Print and shaded views of the part. All mm, measured from the part's lowest x, y and z. A direction names the side the tool comes from. Coordinates: 2 decimals unless noted, no trailing zeros. Write each loop counter-clockwise with the first axis right and the second up, starting at its lowest first coordinate (ties: lowest second). Pieces come first, ordered by that corner, then holes. Notation, with made-up numbers: (-4.5, 84) -> (12.5, 84) arc R13 cw to (12.5, 108) -> close; hole circle Ø3 at (-0.5, 58). An arc over 180 degrees is marked (long way). Write item = value, one per line.
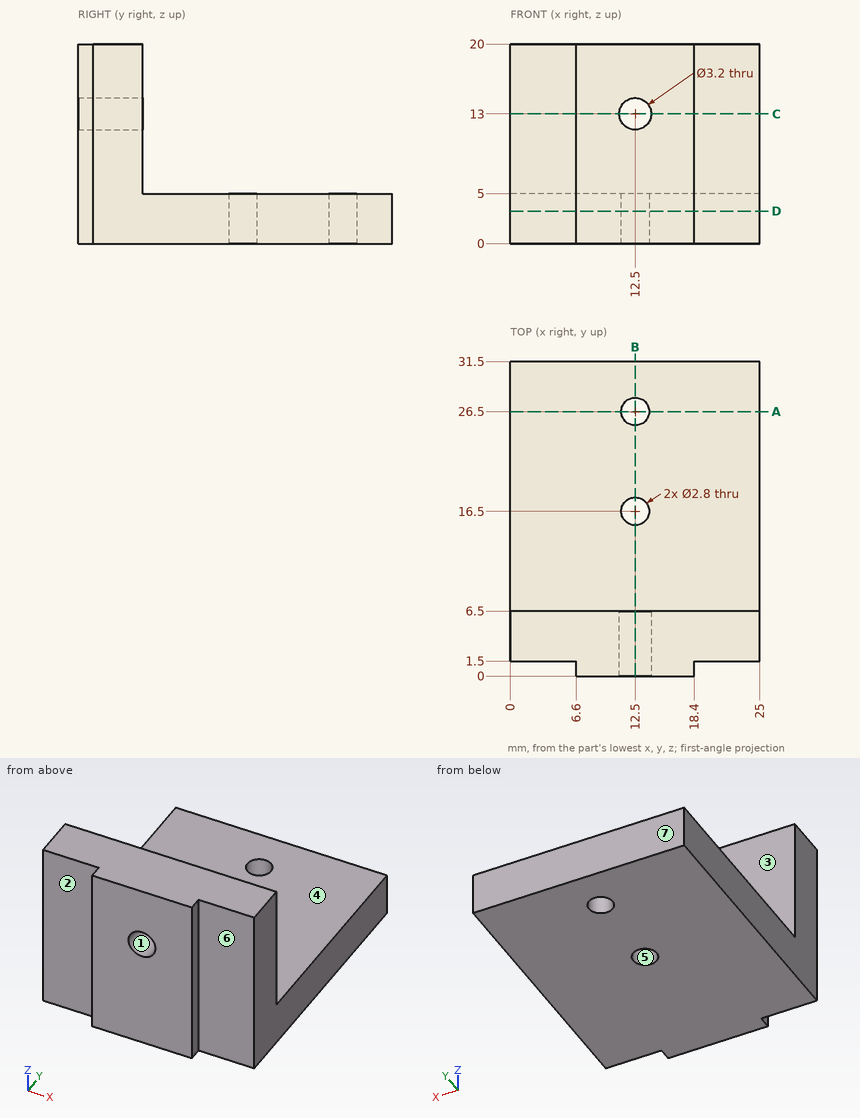
Q1. Saw through at A-A on y = 26.5. Give the cut face in (x, z), and give its area (3 significant figures).
Model answer:
outline = (0, 0) -> (11.1, 0) -> (11.1, 5) -> (0, 5) -> close; (13.9, 0) -> (25, 0) -> (25, 5) -> (13.9, 5) -> close
area = 111 mm²
Q2. Saw through at B-B on x = 12.5. Give the cut face in (y, z).
Model answer:
outline = (0, 0) -> (15.1, 0) -> (15.1, 5) -> (6.5, 5) -> (6.5, 11.4) -> (0, 11.4) -> close; (0, 14.6) -> (6.5, 14.6) -> (6.5, 20) -> (0, 20) -> close; (17.9, 0) -> (25.1, 0) -> (25.1, 5) -> (17.9, 5) -> close; (27.9, 0) -> (31.5, 0) -> (31.5, 5) -> (27.9, 5) -> close
Q3. Saw through at C-C on z = 13. Give the cut face in (x, y), and give its area (3 significant figures).
Model answer:
outline = (0, 1.5) -> (6.6, 1.5) -> (6.6, 0) -> (10.9, 0) -> (10.9, 6.5) -> (0, 6.5) -> close; (14.1, 0) -> (18.4, 0) -> (18.4, 1.5) -> (25, 1.5) -> (25, 6.5) -> (14.1, 6.5) -> close
area = 122 mm²
Q4. Mould opens along Y. For the marked faces 4, 5, 6 and 7 say: released by +Y, released by -Y, zero draft, split by the parting line, or undercut.
Model answer:
face_4 = zero draft
face_5 = undercut
face_6 = released by -Y
face_7 = released by +Y
Q5. Which spindle directions (+Z, -Z, +X, -X, +Y, -Y) get a long thin tool onto all of the face, cutting with end or side? Do the marked faces 1, 2 and 3. Say none if no direction does.
Model answer:
face_1 = +Y, -Y
face_2 = +Z, -Z, -X, -Y
face_3 = +Z, +X, -X, +Y
Q6. Pin check, flat tips, straight feed: pin 1 (4.5 mm diameter, centred on x = 12.5, y = 16.5, fed in from +Z); pin 2 (7.5 mm diameter, centred on x = 10, z = 14.5, fed in from +Y); pin 3 (5.5 mm diameter, centred on x = 22, z = 8, fed in from -Y). Stop position of each tip, or through.
Model answer:
pin_1 = 5
pin_2 = 6.5
pin_3 = 1.5
Q7. Saw through at D-D on z = 3.25. Give the cut face in (x, y).
Model answer:
outline = (0, 1.5) -> (6.6, 1.5) -> (6.6, 0) -> (18.4, 0) -> (18.4, 1.5) -> (25, 1.5) -> (25, 31.5) -> (0, 31.5) -> close; hole circle Ø2.8 at (12.5, 16.5); hole circle Ø2.8 at (12.5, 26.5)
Q8. Probe line 1 (Y direction, x = 12.5, z = 3.5); line 2 (Z direction, x = 12.5, y = 5); line 3 (Y direction, x = 5, z = 17.5). List the from-to ranges inside material, lowest first. Write a range as from..to.
Model answer:
line_1 = 0..15.1, 17.9..25.1, 27.9..31.5
line_2 = 0..11.4, 14.6..20
line_3 = 1.5..6.5
